The model under review builds one solid part; all positions refer to its coordinate system, in mm. A direction names the side the tool comes from. Coordinates: 2 decimals unless noted, no trailing zeros. Loops run counter-clockwise (first coordinate to the right, second up) from the corner with the lowest first, then second, coordinate; pieces in that order, holes last. Notation, with made-up numbers: M 67.25,79.25 L 114.25,79.25 A34 ccw 114.25,118.25 Z; hole C 10,25.25 d10. An arc over 180 degrees is marked long. One line per item, written item: value.
```python
from build123d import *

# Parameters (mm, degrees)
SKETCH1_W           = 100
SKETCH1_H           = 100
SKETCH1_R           = 11
BOSS_EXTRUDE1_DEPTH = 12
SKETCH9_W           = 100
SKETCH9_H           = 50
BOSS_EXTRUDE3_DEPTH = 12
CUT_EXTRUDE3_REACH  = 114.446
SKETCH4_R           = 10.5
CUT_EXTRUDE4_REACH  = 114.446
CUT_EXTRUDE5_REACH  = 114.446
SKETCH6_R           = 26
CUT_EXTRUDE6_REACH  = 114.446
CUT_EXTRUDE7_REACH  = 114.446
SKETCH11_R          = 2.5
CHAMFER1_SIZE       = 10
CUT_EXTRUDE8_REACH  = 114.446
SKETCH12_R          = 3


with BuildPart() as part:
    # Sketch1 → Boss-Extrude1 (new body)
    with BuildSketch(Plane(origin=(0, 0, 0), x_dir=(1, 0, 0), z_dir=(0, 1, 0))):
        Rectangle(SKETCH1_W, SKETCH1_H)
        with Locations(Location((0, 0, 0), (0, 0, 270))):
            Circle(SKETCH1_R, mode=Mode.SUBTRACT)
    extrude(amount=BOSS_EXTRUDE1_DEPTH)

    # Sketch9 → Boss-Extrude3 (add)
    with BuildSketch(Plane(origin=(0, 12, 0), x_dir=(1, 0, 0), z_dir=(0, 1, 0))):
        with Locations((0, -75)):
            Rectangle(SKETCH9_W, SKETCH9_H)
    extrude(amount=-BOSS_EXTRUDE3_DEPTH)

    # Sketch4 → Cut-Extrude3 (cut, up to next)
    with BuildSketch(Plane(origin=(0, 12, 0), x_dir=(1, 0, 0), z_dir=(0, 1, 0)), mode=Mode.PRIVATE) as cut_extrude3_sk1:
        with Locations(Location((-36, -20, 0), (0, 0, 270))):
            Circle(SKETCH4_R)
    cut_extrude3_tool1 = extrude(cut_extrude3_sk1.sketch, amount=-CUT_EXTRUDE3_REACH, mode=Mode.PRIVATE) & part.part
    # Sketch4 → Cut-Extrude3 (cut, up to next)
    with BuildSketch(Plane(origin=(0, 12, 0), x_dir=(1, 0, 0), z_dir=(0, 1, 0)), mode=Mode.PRIVATE) as cut_extrude3_sk2:
        with Locations(Location((36, -20, 0), (0, 0, 270))):
            Circle(SKETCH4_R)
    cut_extrude3_tool2 = extrude(cut_extrude3_sk2.sketch, amount=-CUT_EXTRUDE3_REACH, mode=Mode.PRIVATE) & part.part
    add(cut_extrude3_tool1.solids().sort_by_distance((-36, 12, 20))[0], mode=Mode.SUBTRACT)
    add(cut_extrude3_tool2.solids().sort_by_distance((36, 12, 20))[0], mode=Mode.SUBTRACT)

    # Sketch5 → Cut-Extrude4 (cut, up to next)
    with BuildSketch(Plane(origin=(0, 12, 0), x_dir=(1, 0, 0), z_dir=(0, 1, 0)), mode=Mode.PRIVATE) as cut_extrude4_sk1:
        Polygon((-50, 0), (-32, 0), (-32, 16), (32, 16), (32, 0), (50, 0), (50, 50), (-50, 50), align=None)
    cut_extrude4_tool1 = extrude(cut_extrude4_sk1.sketch, amount=-CUT_EXTRUDE4_REACH, mode=Mode.PRIVATE) & part.part
    add(cut_extrude4_tool1.solids().sort_by_distance((0, 12, -29.37827))[0], mode=Mode.SUBTRACT)

    # Sketch6 → Cut-Extrude5 (cut, up to next)
    with BuildSketch(Plane(origin=(0, 12, 0), x_dir=(1, 0, 0), z_dir=(0, 1, 0)), mode=Mode.PRIVATE) as cut_extrude5_sk1:
        with Locations(Location((-0.234960822, -55, 0), (0, 0, 270))):
            Circle(SKETCH6_R)
    cut_extrude5_tool1 = extrude(cut_extrude5_sk1.sketch, amount=-CUT_EXTRUDE5_REACH, mode=Mode.PRIVATE) & part.part
    add(cut_extrude5_tool1.solids().sort_by_distance((-0.234961, 12, 55))[0], mode=Mode.SUBTRACT)

    # Sketch10 → Cut-Extrude6 (cut, up to next)
    with BuildSketch(Plane(origin=(0, 12, 0), x_dir=(1, 0, 0), z_dir=(0, 1, 0)), mode=Mode.PRIVATE) as cut_extrude6_sk1:
        with BuildLine():
            Line((-10.234960822, -88.541019662), (-10.234960822, -100))
            Line((-10.234960822, -100), (-50, -100))
            Line((-50, -100), (-50, -40))
            Line((-50, -40), (-35.234177398, -54.765822602))
            ThreePointArc((-35.234177398, -54.765822602), (-28.367208461, -75.822503278), (-10.234960822, -88.541019662))
        make_face()
    cut_extrude6_tool1 = extrude(cut_extrude6_sk1.sketch, amount=-CUT_EXTRUDE6_REACH, mode=Mode.PRIVATE) & part.part
    # Sketch10 → Cut-Extrude6 (cut, up to next)
    with BuildSketch(Plane(origin=(0, 12, 0), x_dir=(1, 0, 0), z_dir=(0, 1, 0)), mode=Mode.PRIVATE) as cut_extrude6_sk2:
        with BuildLine():
            Line((9.765039178, -88.541019662), (9.765039178, -100))
            Line((9.765039178, -100), (50, -100))
            Line((50, -100), (50, -40))
            Line((50, -40), (34.764245164, -55.235754836))
            ThreePointArc((34.764245164, -55.235754836), (27.756864791, -76.010894766), (9.765039178, -88.541019662))
        make_face()
    cut_extrude6_tool2 = extrude(cut_extrude6_sk2.sketch, amount=-CUT_EXTRUDE6_REACH, mode=Mode.PRIVATE) & part.part
    # Sketch10 → Cut-Extrude6 (cut, up to next)
    with BuildSketch(Plane(origin=(0, 12, 0), x_dir=(1, 0, 0), z_dir=(0, 1, 0)), mode=Mode.PRIVATE) as cut_extrude6_sk3:
        with BuildLine():
            Line((-0.734960822, -80.995191863), (-0.734960822, -100))
            Line((-0.734960822, -100), (0.265039178, -100))
            Line((0.265039178, -100), (0.265039178, -80.995191863))
            ThreePointArc((0.265039178, -80.995191863), (-0.234960822, -81), (-0.734960822, -80.995191863))
        make_face()
    cut_extrude6_tool3 = extrude(cut_extrude6_sk3.sketch, amount=-CUT_EXTRUDE6_REACH, mode=Mode.PRIVATE) & part.part
    add(cut_extrude6_tool1.solids().sort_by_distance((-35.978986, 12, 79.410224))[0], mode=Mode.SUBTRACT)
    add(cut_extrude6_tool2.solids().sort_by_distance((35.780347, 12, 79.379296))[0], mode=Mode.SUBTRACT)
    add(cut_extrude6_tool3.solids().sort_by_distance((-0.234961, 12, 90.499199))[0], mode=Mode.SUBTRACT)

    # Sketch11 → Cut-Extrude7 (cut, up to next)
    with BuildSketch(Plane(origin=(0, 12, 0), x_dir=(1, 0, 0), z_dir=(0, 1, 0)), mode=Mode.PRIVATE) as cut_extrude7_sk1:
        with Locations(Location((-16.5, 0, 0), (0, 0, 270))):
            Circle(SKETCH11_R)
    cut_extrude7_tool1 = extrude(cut_extrude7_sk1.sketch, amount=-CUT_EXTRUDE7_REACH, mode=Mode.PRIVATE) & part.part
    # Sketch11 → Cut-Extrude7 (cut, up to next)
    with BuildSketch(Plane(origin=(0, 12, 0), x_dir=(1, 0, 0), z_dir=(0, 1, 0)), mode=Mode.PRIVATE) as cut_extrude7_sk2:
        with Locations(Location((16.5, 0, 0), (0, 0, 270))):
            Circle(SKETCH11_R)
    cut_extrude7_tool2 = extrude(cut_extrude7_sk2.sketch, amount=-CUT_EXTRUDE7_REACH, mode=Mode.PRIVATE) & part.part
    add(cut_extrude7_tool1.solids().sort_by_distance((-16.5, 12, 0))[0], mode=Mode.SUBTRACT)
    add(cut_extrude7_tool2.solids().sort_by_distance((16.5, 12, 0))[0], mode=Mode.SUBTRACT)

    # Chamfer1
    chamfer1_edges = [part.edges().sort_by_distance(p)[0] for p in [
        (32, 6, -16),
        (-32, 6, -16),
    ]]
    chamfer(chamfer1_edges, length=CHAMFER1_SIZE)

    # Sketch12 → Cut-Extrude8 (cut, up to next)
    with BuildSketch(Plane(origin=(0, 12, 0), x_dir=(1, 0, 0), z_dir=(0, 1, 0)), mode=Mode.PRIVATE) as cut_extrude8_sk1:
        with Locations(Location((15, -20, 0), (0, 0, 270))):
            Circle(SKETCH12_R)
    cut_extrude8_tool1 = extrude(cut_extrude8_sk1.sketch, amount=-CUT_EXTRUDE8_REACH, mode=Mode.PRIVATE) & part.part
    # Sketch12 → Cut-Extrude8 (cut, up to next)
    with BuildSketch(Plane(origin=(0, 12, 0), x_dir=(1, 0, 0), z_dir=(0, 1, 0)), mode=Mode.PRIVATE) as cut_extrude8_sk2:
        with Locations(Location((-15, -20, 0), (0, 0, 270))):
            Circle(SKETCH12_R)
    cut_extrude8_tool2 = extrude(cut_extrude8_sk2.sketch, amount=-CUT_EXTRUDE8_REACH, mode=Mode.PRIVATE) & part.part
    add(cut_extrude8_tool1.solids().sort_by_distance((15, 12, 20))[0], mode=Mode.SUBTRACT)
    add(cut_extrude8_tool2.solids().sort_by_distance((-15, 12, 20))[0], mode=Mode.SUBTRACT)


solid = part.part
```
(1) Draft analysis for pull direction X (two halves, no side actions). For faces 1 (the face through (-17.93, 6.08, 19.35)), 2 (the face through (-1, 12, 28)), 3 (the face through (32, 6, -3)), 4 (the face through (18.61, 6.08, 1.34)), state which applies: pulls with the +X half, pulls with the -X half, needs draft (parallel to the pull), parting line crosses it, or undercut.
Checks:
face 1: undercut
face 2: needs draft
face 3: pulls with the +X half
face 4: undercut
(2) Add section D-D on x = -16.5. State the section outline as (y, z) points.
Checks:
outline: M 0,-16 L 12,-16 L 12,-2.5 L 0,-2.5 Z; M 0,2.5 L 12,2.5 L 12,17.4 L 0,17.4 Z; M 0,22.6 L 12,22.6 L 12,34.72 L 0,34.72 Z; M 0,75.28 L 12,75.28 L 12,85.99 L 0,85.99 Z
(3) Insertion check: pin 1 Ø1.5 at (y, z) = (8.5, 43.5) entering from -X; pin 2 Ø6 at (y, z) = (5.5, 86.5) entering from +X; pin 3 Ø1.8 at (y, z) = (8.5, -3) entering from +X. Each pin has a flat end and moves straight along its axis. Give the tip position at first contact, or say it passes through.
Checks:
pin 1: x = -47.25
pin 2: x = 20.08
pin 3: x = 32
(4) Tool access review of faces 5 (the face through (-32, 6, -3)), 6 (the face through (-1, 0, 28)), 7 (the face through (41, 6, 0)), 8 (the face through (-0.735, 6, 90)), 9 (the face through (9.765, 6, 94)): name each direction out of +Z, -Z, +X, -X, +Y, -Y from which nothing blocks a thin tool from reaching the whole face with its end or side.
Checks:
face 5: -Z, -X, +Y, -Y
face 6: +Z, -Z, +X, -X, -Y
face 7: -Z, +X, +Y, -Y
face 8: +Z, +Y, -Y
face 9: +Z, +X, +Y, -Y
(5) Add section A-A on x = 36. State the section outline as (y, z) points, then the cut area to 3 significant figures.
Checks:
outline: M 0,0 L 12,0 L 12,9.5 L 0,9.5 Z; M 0,30.5 L 12,30.5 L 12,54 L 0,54 Z
area: 396 mm^2
(6) Add section B-B on z = 59.5. State the section outline as (x, y) points, then the cut area to 3 significant figures.
Checks:
outline: M -34.94,0 L -25.84,0 L -25.84,12 L -34.94,12 Z; M 25.37,0 L 34.47,0 L 34.47,12 L 25.37,12 Z
area: 218 mm^2
(7) To check wall thickness, follow L1, parallel to X at y = 6, z = 20; L2, parallel to X at y = 10.5, z = 13; L3, parallel to X at y = 10.5, z = 24. State the ranges of each line that lie inside material, in increasing order. Write a range as [from, to].
Checks:
L1: [-50, -46.5], [-25.5, -18], [-12, 12], [18, 25.5], [46.5, 50]
L2: [-50, -43.83], [-28.17, 28.17], [43.83, 50]
L3: [-50, -45.71], [-26.29, 26.29], [45.71, 50]
(8) Add section C-C on y = 8.75. State the section outline as (x, z) points.
Checks:
outline: M -50,0 L -32,0 L -32,-6 L -22,-16 L 22,-16 L 32,-6 L 32,0 L 50,0 L 50,40 L 34.76,55.24 A35 ccw 9.77,88.54 L 9.77,100 L 0.27,100 L 0.27,81 A26 cw long -0.73,81 L -0.73,100 L -10.23,100 L -10.23,88.54 A35 ccw -35.23,54.77 L -50,40 Z; hole C -36,20 d21; hole C -16.5,0 d5; hole C -15,20 d6; hole C 0,0 d22; hole C 15,20 d6; hole C 16.5,0 d5; hole C 36,20 d21
